from build123d import *

# Parameters (mm, degrees)
ESQUISSE2_W        = 90
ESQUISSE2_H        = 42
BOSS_EXTRU_1_DEPTH = 50
CHANFREIN1_SIZE    = 1
EXTRU_MINCE1_DEPTH = 3


with BuildPart() as part:
    # Esquisse2 → Boss.-Extru.1 (new body)
    with BuildSketch(Plane(origin=(0, 0, 0), x_dir=(1, 0, 0), z_dir=(0, 1, 0))):
        Rectangle(ESQUISSE2_W, ESQUISSE2_H)
    extrude(amount=BOSS_EXTRU_1_DEPTH)

    # Chanfrein1
    chanfrein1_edges = [part.edges().sort_by_distance(p)[0] for p in [
        (-45, 50, 0),
        (0, 50, 21),
        (45, 50, 0),
        (0, 0, 21),
        (-45, 0, 0),
        (0, 0, -21),
        (45, 0, 0),
        (45, 25, 21),
        (-45, 25, 21),
        (-45, 25, -21),
        (45, 25, -21),
        (0, 50, -21),
    ]]
    chamfer(chanfrein1_edges, length=CHANFREIN1_SIZE)

    # Esquisse5 → Extru.-Mince1 (add, symmetric)
    with BuildSketch(Plane.XY.offset(13)):
        Polygon((-24.585, 50), (-24.585, 53.6815593), (-17.428488481, 55.599140782), (-17.643308289, 56.400859218), (-25.415, 54.3184407), (-25.415, 50), align=None)
    extru_mince1 = extrude(amount=EXTRU_MINCE1_DEPTH, both=True)

    # Symétrie1: Extru.-Mince1 across plane
    add(extru_mince1.mirror(Plane.XY))


solid = part.part
The model under review builds one solid part; all positions refer to its coordinate system, in mm. A direction names the side the tool comes from. Give positions to 0.01 mm unless a question says otherwise; leave off trailing zeros. Order: outer loops, then holes, each group sorted by start corner. A loop starts at its lowest first (then second) coordinate and runs counter-clockwise, first axis right, second up. Notation, with made-up numbers: M -12,-35 L 36,-35 A31 cw 36,-1 Z; hole C 89,82.5 d5. An arc over 180 degrees is marked long. One line per question, with ' | ' between items. Start each with the question number.
1) For faces 4 (the face through (-22.6, 54.4, -10)), 5 (the face through (-24.585, 52, 13)), 6 (the face through (-45, 25, 0)), 7 (the face through (-22.6, 54.4, -16)), 8 (the face through (-25.415, 52, -13)), list the 3-axis set-ups (+Z, -Z, +X, -X, +Y, -Y) from which the entire face can be reached by the end or side of a thin tool; tool diameter is ignored.
2) Consider section D-D, the plane x = 35.5. Give the boundary of the cut face in (y, z).
3) Consider section B-B, the plane z = -17. Give the boundary of the cut face in (x, y), then the cut area to 3 significant figures.
4) Mouldability with a two-part tool opening along Y and no side actions: class faces 1 (the face through (-21.475, 55.374, -13.042)), 2 (the face through (-22.6, 54.4, 16)), 3 (the face through (-24.585, 52, -13)) as pulls with the +Y half, pulls with the -Y half, needs draft (parallel to the pull), parting line crosses it, or undercut.
5) Consider section C-C, the plane x = -19.5. Give the boundary of the cut face in (y, z).
6) Consider section A-A, the plane y = 51. Give the boundary of the cut face in (x, z) (3 decimals).
7) Clearance check with flat-ended pins moving along their axes: P1, Ø5, axis at x = -21, y = 53.5, coming from the -Z side; P2, Ø1.1, axis at y = 52, z = -14.5, coming from the +X side (3 decimals); P3, Ø5, axis at x = -20.5, y = 54, coming from the +Z side. State where each tip first meets the part, or that it passes through.
8) Wall thickness on L1, parallel to Y at x = -29, z = 14.5; L2, parallel to X at y = 53, z = -10.5 (3 decimals); L3, parallel to Y at x = -20, z = 14: over which ranges is each line inside the solid? List them lowest first. Write a range as from..to.
Found:
1) face 4: +X, -X, +Y | face 5: +Z, -Z, +X | face 6: +Z, -Z, -X, +Y, -Y | face 7: -Z, +X, -X, +Y | face 8: +Z, -Z, -X, +Y
2) outline: M 0,-20 L 1,-21 L 49,-21 L 50,-20 L 50,20 L 49,21 L 1,21 L 0,20 Z
3) outline: M -45,1 L -44,0 L 44,0 L 45,1 L 45,49 L 44,50 L -44,50 L -45,49 Z | area: 4,500 mm²
4) face 1: pulls with the +Y half | face 2: needs draft | face 3: undercut
5) outline: M 0,-20 L 1,-21 L 49,-21 L 50,-20 L 50,20 L 49,21 L 1,21 L 0,20 Z; M 55.04,-16 L 55.9,-16 L 55.9,-10 L 55.04,-10 Z; M 55.04,10 L 55.9,10 L 55.9,16 L 55.04,16 Z
6) outline: M -25.415,-16 L -24.585,-16 L -24.585,-10 L -25.415,-10 Z; M -25.415,10 L -24.585,10 L -24.585,16 L -25.415,16 Z
7) P1: stops at z = -16 | P2: stops at x = -24.585 | P3: stops at z = 16
8) L1: y = 0..50 | L2: x = -25.415..-24.585 | L3: y = 0..50, 54.91..55.77
